Model file for the job. Use its own axes, mm. Face numbers are marked on the shaded views. Give positions to 0.01 mm unless a question says otherwise; leave off trailing zeros. Write each loop counter-clockwise with the first axis right and the second up, starting at its lowest first coordinate (ties: lowest second). Pieces come first, ordered by that corner, then holes. Notation, with made-up numbers: (30, 59.5) - (42, 59.5) arc R29 cw to (42, 93.5) - close; hole circle Ø4 at (-3, -17). An arc over 180 degrees is marked (long way). One line per item, written item: value. Start each with the question number.
(1) Mould opens along X. For the marked faces 1, 2, 3 and 4 say: pulls with the +X half, pulls with the -X half, needs draft (parallel to the pull), parting line crosses it, or undercut.
(2) Probe L1, parallel to X at y = 8, z = 4.35; L2, parallel to Y at x = 0, z = 2.15; L3, parallel to Y at x = 13, z = 3.2. List the from-to ranges inside material, lowest first.
(3) Cut at C-C, the plane y = -6.75. List the corners of the cut face in (x, z), and give its area (3 significant figures).
(4) Drop flat-ended pins along their axis: P1, Ø2, axis at y = 4, z = 3.5, coming from the +X side; P2, Ø1.5, axis at x = 7, z = 0.5, coming from the -Y side; P3, Ø3, axis at y = 10.5, z = 3.5, coming from the -X side. Give the stop position or say it passes through.
(5) Cut at B-B, the plane x = 0. List the corners of the cut face in (y, z).
(6) Cut at A-A, the plane y = 0. List the corners of the cut face in (x, z), and give its area (3 significant figures).
(7) Cut at D-D, the plane x = -4. List the corners of the cut face in (y, z).
Autodesk Inventor part; units mm, degrees
ref_plane "YZ Plane" through (0, 0, 0) normal (1, 0, 0) x (0, 1, 0)
ref_plane "XZ Plane" through (0, 0, 0) normal (0, 1, 0) x (-1, 0, 0)
ref_plane "XY Plane" through (0, 0, 0) normal (0, 0, 1) x (1, 0, 0)
sketch "スケッチ1" plane through (0, 0, 0) normal (0, 0, 1) x (1, 0, 0)
  circle A0 centre (0, 0) radius 17.5
  dimension "d0" = 35
extrude "押し出し1" add sketch "スケッチ1" along normal blind 5
sketch "スケッチ2" plane through (0, 0, 5) normal (0, 0, 1) x (1, 0, 0)
  circle A0 centre (0, 0) radius 13.5
  point P0 (0, 13.5)
  point P1 (-11.6913, 6.75)
  point P2 (-11.6913, -6.75)
  point P3 (0, -13.5)
  point P4 (11.6913, -6.75)
  point P5 (11.6913, 6.75)
  dimension "d3" = 27
  dimension "d6" = 360
hole "穴1" at (0, 13.5, 5) at (-11.6913, 6.75, 5) at (-11.6913, -6.75, 5) at (0, -13.5, 5) at (11.6913, -6.75, 5) at (11.6913, 6.75, 5) direction (0, 0, -1) diameter 3.2 end through all
sketch "スケッチ3" plane through (0, 0, 0) normal (0, 0, -1) x (-1, 0, 0)
  circle A0 centre (0, 0) radius 10
  dimension "d15" = 20
extrude "押し出し2" cut sketch "スケッチ3" against normal blind 5
properties part number "servohorn_forR0" material "アルミニウム 6061"
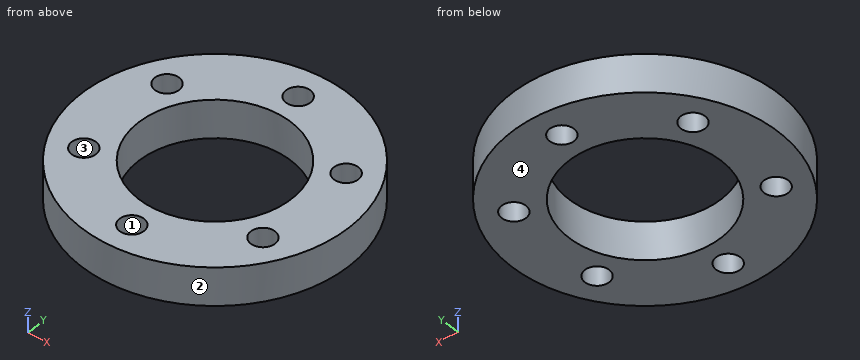
Answers follow:
1. face 1: undercut
1. face 2: parting line crosses it
1. face 3: undercut
1. face 4: needs draft
2. L1: x = -15.56 to -12.69, -10.69 to -6, 6 to 10.69, 12.69 to 15.56
2. L2: y = -17.5 to -15.1, -11.9 to -10, 10 to 11.9, 15.1 to 17.5
2. L3: y = -11.72 to -7.67, -5.83 to 5.83, 7.67 to 11.72
3. outline: (-16.15, 0) - (-13.29, 0) - (-13.29, 5) - (-16.15, 5) - close; (-10.09, 0) - (-7.38, 0) - (-7.38, 5) - (-10.09, 5) - close; (7.38, 0) - (10.09, 0) - (10.09, 5) - (7.38, 5) - close; (13.29, 0) - (16.15, 0) - (16.15, 5) - (13.29, 5) - close
3. area: 55.7 mm²
4. P1: stops at x = 17.24
4. P2: stops at y = -16.35
4. P3: stops at x = -15.01
5. outline: (-17.5, 0) - (-15.1, 0) - (-15.1, 5) - (-17.5, 5) - close; (-11.9, 0) - (-10, 0) - (-10, 5) - (-11.9, 5) - close; (10, 0) - (11.9, 0) - (11.9, 5) - (10, 5) - close; (15.1, 0) - (17.5, 0) - (17.5, 5) - (15.1, 5) - close
6. outline: (-17.5, 0) - (-10, 0) - (-10, 5) - (-17.5, 5) - close; (10, 0) - (17.5, 0) - (17.5, 5) - (10, 5) - close
6. area: 75.0 mm²
7. outline: (-17.04, 0) - (-9.17, 0) - (-9.17, 5) - (-17.04, 5) - close; (9.17, 0) - (17.04, 0) - (17.04, 5) - (9.17, 5) - close
